Source: CAD feature listing. Evaluate the final solid. Frame: model axes, mm. A direction names the side the tool comes from. Coordinates: 2 decimals unless noted, no trailing zeros. Loops run counter-clockwise (first coordinate to the right, second up) from the corner with the lowest first, then second, coordinate; pieces in that order, holes last. Notation, with made-up numbers: (-22.5, 5) - (-5.5, 5) arc R10 cw to (-5.5, 22) - close; hole circle Ø10 at (7, 80.5). An arc over 180 degrees is marked (long way). Use one line per item in the form item = value. Start each with the question number.
from build123d import *

# Parameters (mm, degrees)
F0_W     = 15.0114
F0_H     = 19.8755
F0_W_2   = 7.2136
F0_H_2   = 10.287
F2_R     = 1.5875
F3_SIZE2 = 1.5748
F3_SIZE  = 6.35


with BuildPart() as f1:
    # F0 (on Right) → F1 (revolve)
    with BuildSketch(Plane.YZ):
        with Locations((14.7193, 15.46225)):
            Rectangle(F0_W, F0_H)
        with Locations((3.6068, 15.46225)):
            Rectangle(F0_W_2, F0_H)
        with Locations((3.6068, 30.5435)):
            Rectangle(F0_W_2, F0_H_2)
    revolve(axis=Axis((0, 11.1125, 0), (0, 1, 0)))

    # F2
    f2_edges = [f1.edges().sort_by_distance(p)[0] for p in [
        (0, 7.2136, -25.4),
    ]]
    fillet(f2_edges, radius=F2_R)

    # F3
    f3_edges = [f1.edges().sort_by_distance(p)[0] for p in [
        (0, 22.225, -25.4),
    ]]
    chamfer(f3_edges, length=F3_SIZE, length2=F3_SIZE2)


solid = f1.part
(1) Cut plane C-C, the plane y = 11. Output: boundary loops of the cut face in (x, z), plus the area to 3 significant figures.
(2) Cut plane B-B, the plane z = 0. Output: boundary loops of the cut face in (x, y) (1 decimal).
(3) Cut plane D-D, the plane z = 29.5. Output: boundary loops of the cut face in (x, y), plus the area to 3 significant figures.
(4) Material intervals for line 1 (X direction, y = 10.25, z = 0); line 2 (X direction, y = 4.5, z = 0); line 3 (Y direction, x = -20.5, z = -24), sorted ascending.
(5) Cut plane A-A, the plane x = 0. Output: boundary loops of the cut face in (y, z) (1 decimal).
(6) Contact query for flat-ended pins moving along their axis: pin 1 (1.5 mm diameter, centred on y = 12, z = 3, fed in from -X); pin 2 (6 mm diameter, centred on x = -24, y = 17, fed in from +Z); pin 3 (1.5 mm diameter, centred on x = 12, y = 15.5, fed in from +Z); pin 4 (6.5 mm diameter, centred on x = 0, z = 0, fed in from +Y). Output: stop coordinate, or through.
(7) Access query for faces 4 (the face through (0, 22.225, 6)), 5 (the face through (27, 7.214, -5)). Directions: +Z, -Z, +X, -X, +Y, -Y. A direction counts if a zero-diameter tool reaches every point of the face in a straight line with its end or side. Return the directions, or none.
(8) Mould query, pull axis Z, two halves, no side actions, for faces 1 (the face through (30.09, 3.66, 19.19)), 2 (the face through (5.477, 11.268, -0.719)), 3 (the face through (-7, 0, 0)). Classes: +Z half, -Z half, draft (parallel to the pull), parting line (faces both ways), or undercut.
Recorded:
q1.outline = circle Ø50.8 at (0, 0); hole circle Ø11.05 at (0, 0)
q1.area = 1,930 mm²
q2.outline = (-35.7, 0) - (-5.5, 0) - (-5.5, 22.2) - (-23.8, 22.2) - (-25.4, 15.9) - (-25.4, 8.8) arc R1.6 cw to (-27, 7.2) - (-35.7, 7.2) - close; (5.5, 0) - (35.7, 0) - (35.7, 7.2) - (27, 7.2) arc R1.6 cw to (25.4, 8.8) - (25.4, 15.9) - (23.8, 22.2) - (5.5, 22.2) - close
q3.outline = (-20.08, 0) - (20.08, 0) - (20.08, 7.21) - (-20.08, 7.21) - close
q3.area = 290 mm²
q4.line_1 = -25.4 to -5.52, 5.52 to 25.4
q4.line_2 = -35.69 to -5.52, 5.52 to 35.69
q4.line_3 = 0 to 7.21
q5.outline = (0, -35.7) - (7.2, -35.7) - (7.2, -27) arc R1.6 cw to (8.8, -25.4) - (15.9, -25.4) - (22.2, -23.8) - (22.2, -5.5) - (0, -5.5) - close; (0, 5.5) - (22.2, 5.5) - (22.2, 23.8) - (15.9, 25.4) - (8.8, 25.4) arc R1.6 cw to (7.2, 27) - (7.2, 35.7) - (0, 35.7) - close
q6.pin_1 = -25.3
q6.pin_2 = 13.98
q6.pin_3 = 22.77
q6.pin_4 = through
q7.face_4 = +Z, -Z, +X, -X, +Y
q7.face_5 = +Y
q8.face_1 = parting line
q8.face_2 = undercut
q8.face_3 = draft
